Read the model definition and answer for the solid it produces. Units are mm, in the model's axes. Coordinates: 2 decimals unless noted, no trailing zeros. Loops run counter-clockwise (first coordinate to the right, second up) from the corner with the lowest first, then second, coordinate; pieces in that order, holes last. Notation, with made-up numbers: (78, -39.5) - (85, -39.5) arc R17 cw to (85, -14.5) - close; hole circle Ø6 at (38.5, -38). An arc over 180 degrees is marked (long way). One line per item, written item: value. Start each with the question number.
from build123d import *

# Parameters (mm, degrees)
SKETCH1_R           = 2.5
BOSS_EXTRUDE1_DEPTH = 3


with BuildPart() as part:
    # Sketch1 → Boss-Extrude1 (new body)
    with BuildSketch(Plane.XY):
        with BuildLine():
            Line((167.77621964, -174.96032759), (287.77621964, -174.96032759))
            ThreePointArc((287.77621964, -174.96032759), (308.989423075, -166.173531026), (317.77621964, -144.96032759))
            Line((317.77621964, -144.96032759), (317.77621964, -92.46032759))
            ThreePointArc((317.77621964, -92.46032759), (325.27621964, -84.96032759), (317.77621964, -77.46032759))
            Line((317.77621964, -77.46032759), (317.77621964, -24.96032759))
            ThreePointArc((317.77621964, -24.96032759), (308.989423075, -3.747124154), (287.77621964, 5.03967241))
            Line((287.77621964, 5.03967241), (167.77621964, 5.03967241))
            ThreePointArc((167.77621964, 5.03967241), (146.563016204, -3.747124154), (137.77621964, -24.96032759))
            Line((137.77621964, -24.96032759), (137.77621964, -77.46032759))
            ThreePointArc((137.77621964, -77.46032759), (130.27621964, -84.96032759), (137.77621964, -92.46032759))
            Line((137.77621964, -92.46032759), (137.77621964, -144.96032759))
            ThreePointArc((137.77621964, -144.96032759), (146.563016204, -166.173531026), (167.77621964, -174.96032759))
        make_face()
        with Locations((317.77621964, -84.96032759)):
            Circle(SKETCH1_R, mode=Mode.SUBTRACT)
        with Locations((137.77621964, -84.96032759)):
            Circle(SKETCH1_R, mode=Mode.SUBTRACT)
        with BuildLine():
            Line((226.284678956, -14.96032759), (167.784678956, -14.96032759))
            ThreePointArc((167.784678956, -14.96032759), (160.713611144, -17.889259778), (157.784678956, -24.96032759))
            Line((157.784678956, -24.96032759), (150.784678956, -24.96032759))
            Line((150.784678956, -24.96032759), (150.784678956, -74.96032759))
            Line((150.784678956, -74.96032759), (157.784678956, -74.96032759))
            Line((157.784678956, -74.96032759), (157.784678956, -83.46032759))
            Line((157.784678956, -83.46032759), (147.784678956, -83.46032759))
            Line((147.784678956, -83.46032759), (147.784678956, -86.46032759))
            Line((147.784678956, -86.46032759), (157.784678956, -86.46032759))
            Line((157.784678956, -86.46032759), (297.784678956, -86.46032759))
            Line((297.784678956, -86.46032759), (307.784678956, -86.46032759))
            Line((307.784678956, -86.46032759), (307.784678956, -83.46032759))
            Line((307.784678956, -83.46032759), (297.784678956, -83.46032759))
            Line((297.784678956, -83.46032759), (297.784678956, -74.96032759))
            Line((297.784678956, -74.96032759), (304.784678956, -74.96032759))
            Line((304.784678956, -74.96032759), (304.784678956, -24.96032759))
            Line((304.784678956, -24.96032759), (297.784678956, -24.96032759))
            ThreePointArc((297.784678956, -24.96032759), (294.855746768, -17.889259778), (287.784678956, -14.96032759))
            Line((287.784678956, -14.96032759), (229.284678956, -14.96032759))
            Line((229.284678956, -14.96032759), (226.284678956, -14.96032759))
        make_face(mode=Mode.SUBTRACT)
        with BuildLine():
            Line((246.743573739, -106.823862957), (246.743573739, -148.163900951))
            ThreePointArc((246.743573739, -148.163900951), (255.784678956, -157.205006168), (264.825784173, -148.163900951))
            Line((264.825784173, -148.163900951), (264.825784173, -106.823862957))
            ThreePointArc((264.825784173, -106.823862957), (255.784678956, -97.78275774), (246.743573739, -106.823862957))
        make_face(mode=Mode.SUBTRACT)
        with BuildLine():
            Line((236.825784173, -106.823862957), (236.825784173, -148.163900951))
            ThreePointArc((236.825784173, -148.163900951), (227.784678956, -157.205006168), (218.743573739, -148.163900951))
            Line((218.743573739, -148.163900951), (218.743573739, -106.823862957))
            ThreePointArc((218.743573739, -106.823862957), (227.784678956, -97.78275774), (236.825784173, -106.823862957))
        make_face(mode=Mode.SUBTRACT)
        with BuildLine():
            Line((274.743573739, -106.823862957), (274.743573739, -148.163900951))
            ThreePointArc((274.743573739, -148.163900951), (283.784678956, -157.205006168), (292.825784173, -148.163900951))
            Line((292.825784173, -148.163900951), (292.825784173, -106.823862957))
            ThreePointArc((292.825784173, -106.823862957), (283.784678956, -97.78275774), (274.743573739, -106.823862957))
        make_face(mode=Mode.SUBTRACT)
        with BuildLine():
            Line((190.743573739, -106.823862957), (190.743573739, -148.163900951))
            ThreePointArc((190.743573739, -148.163900951), (199.784678956, -157.205006168), (208.825784173, -148.163900951))
            Line((208.825784173, -148.163900951), (208.825784173, -106.823862957))
            ThreePointArc((208.825784173, -106.823862957), (199.784678956, -97.78275774), (190.743573739, -106.823862957))
        make_face(mode=Mode.SUBTRACT)
        with BuildLine():
            Line((162.743573739, -106.823862957), (162.743573739, -148.163900951))
            ThreePointArc((162.743573739, -148.163900951), (171.784678956, -157.205006168), (180.825784173, -148.163900951))
            Line((180.825784173, -148.163900951), (180.825784173, -106.823862957))
            ThreePointArc((180.825784173, -106.823862957), (171.784678956, -97.78275774), (162.743573739, -106.823862957))
        make_face(mode=Mode.SUBTRACT)
    extrude(amount=BOSS_EXTRUDE1_DEPTH)


solid = part.part
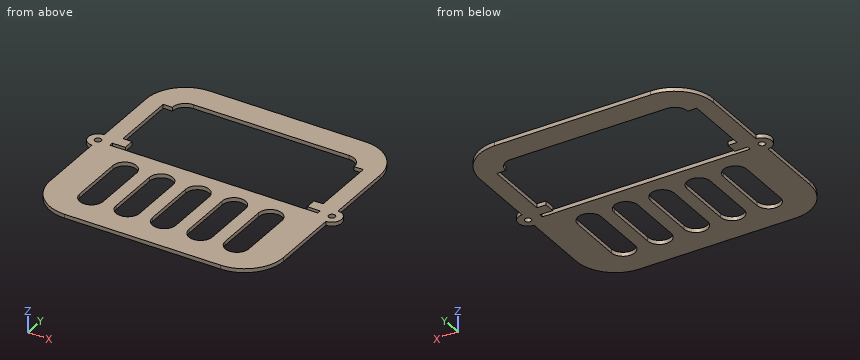
1) Section D-D, the plane z = 1.6 is taken. State how many separate pieces and enclosed holes the cut face has, and give its area (3 significant figures).
2) Flat-ended cylindrical pins translate along their axes: P1, Ø0.9, axis at y = -137.5, z = 1, coming from the -X side; P2, Ø1.5, axis at y = -117.5, z = 1, coming from the +X side; P3, Ø0.9, axis at x = 150.5, z = 1.5, coming from the -Y side; P4, Ø12, axis at x = 169.5, y = -135, coming from the +Z side. Find the tip coordinate at first contact, or state that the pin passes through.
3) Section C-C, the plane x = 277.5 is taken. Determine the outline of the cut face in (y, z), and give its area (3 significant figures).
4) Section B-B, the plane x = 187.5 is taken. Determine the outline of the cut face in (y, z), and give its area (4 significant figures).
5) Section A-A, the plane y = -133 is taken. Determine the outline of the cut face in (x, z).
6) Straight lines are drawn through the part: L1, parallel to Y at x = 255.5, z = 0.65; L2, parallel to X at y = -122.5, z = 1.6; L3, parallel to X at y = -48.5, z = 2.7. For each, find the intervals that lie inside material, in ascending order.
Answer below:
1. separate pieces: 1
1. enclosed holes: 8
1. area: 16,000 mm2
2. P1: x = 137.78
2. P2: x = 317.78
2. P3: y = -169.8
2. P4: through
3. outline: (-174.96, 0) - (-154.66, 0) - (-154.66, 3) - (-174.96, 3) - close; (-100.32, 0) - (-86.46, 0) - (-86.46, 3) - (-100.32, 3) - close; (-14.96, 0) - (5.04, 0) - (5.04, 3) - (-14.96, 3) - close
3. area: 162 mm2
4. outline: (-174.96, 0) - (-86.46, 0) - (-86.46, 3) - (-174.96, 3) - close; (-14.96, 0) - (5.04, 0) - (5.04, 3) - (-14.96, 3) - close
4. area: 325.5 mm2
5. outline: (137.78, 0) - (162.74, 0) - (162.74, 3) - (137.78, 3) - close; (180.83, 0) - (190.74, 0) - (190.74, 3) - (180.83, 3) - close; (208.83, 0) - (218.74, 0) - (218.74, 3) - (208.83, 3) - close; (236.83, 0) - (246.74, 0) - (246.74, 3) - (236.83, 3) - close; (264.83, 0) - (274.74, 0) - (274.74, 3) - (264.83, 3) - close; (292.83, 0) - (317.78, 0) - (317.78, 3) - (292.83, 3) - close
6. L1: -174.96 to -157.2, -97.79 to -86.46, -14.96 to 5.04
6. L2: 137.78 to 162.74, 180.83 to 190.74, 208.83 to 218.74, 236.83 to 246.74, 264.83 to 274.74, 292.83 to 317.78
6. L3: 137.78 to 150.78, 304.78 to 317.78
